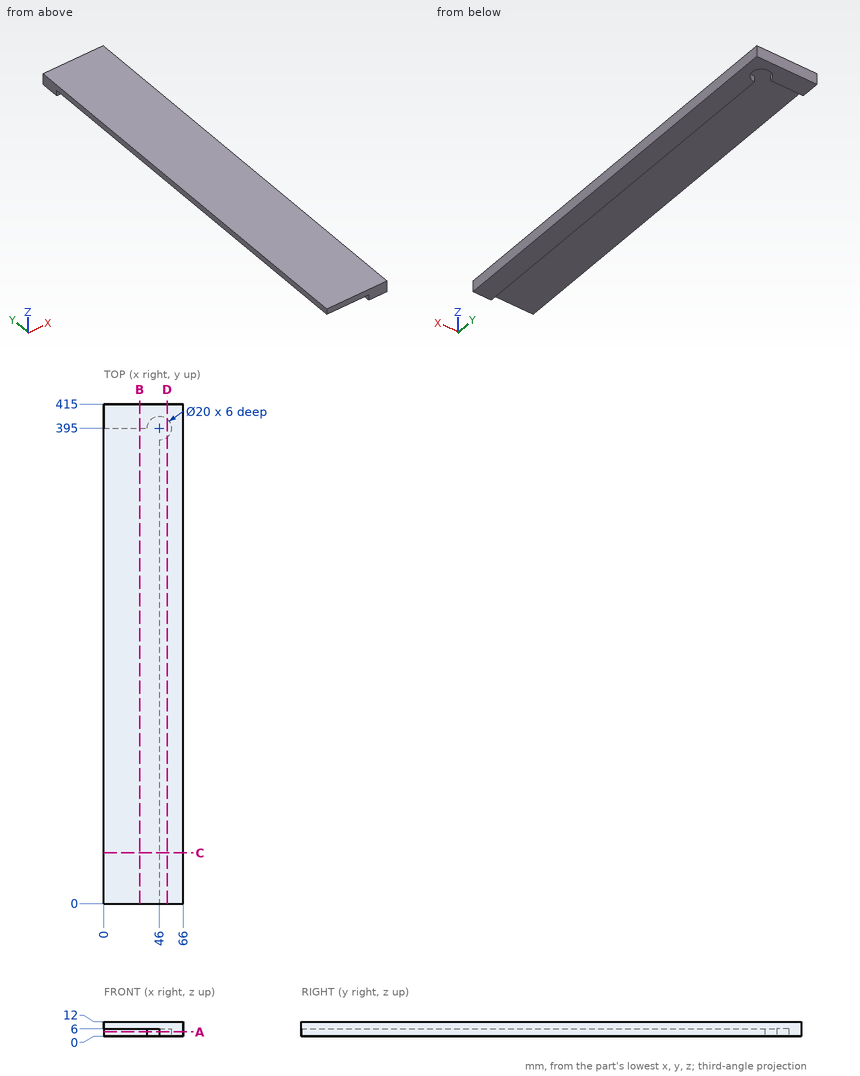
Answer from the drawing. Dimensions are ordinates in mm from the lowest x, y and z of the part. Coordinates: 2 decimals unless noted, no trailing zeros. Loops run counter-clockwise (first coordinate to the right, second up) from the corner with the lowest first, then second, coordinate; pieces in that order, holes last. Notation, with made-up numbers: (89.25, 19.5) -> (126.25, 19.5) arc R22 cw to (126.25, 33.5) -> close; hole circle Ø3 at (76.5, -3). An arc over 180 degrees is marked (long way). Answer as CSV lines item,"result".
Q1. The part is cut by section B-B on x = 29.5. Write down the section's boundary in (y, z), and give its area (3 significant figures).
Findings:
outline,"(0, 6) -> (395, 6) -> (395, 0) -> (415, 0) -> (415, 12) -> (0, 12) -> close"
area,"2,610 mm²"
Q2. Find the intervals of material crossed by probe 1 along X at (y, z) = (171, 3.75); probe 2 along Z at (x, y) = (45, 150); probe 3 along Y at (x, z) = (14.5, 1), in increasing order.
Findings:
probe 1,"x = 46 to 66"
probe 2,"z = 6 to 12"
probe 3,"y = 395 to 415"
Q3. The part is cut by section D-D on x = 52.5. Write down the section's boundary in (y, z).
Findings:
outline,"(0, 0) -> (387.4, 0) -> (387.4, 6) -> (402.6, 6) -> (402.6, 0) -> (415, 0) -> (415, 12) -> (0, 12) -> close"
Q4. Each of these flat-tipped pins is pushed along its axis until it touches: pin 1 (5 mm diameter, centred on y = 221.5, z = 3, fed in from -X); pin 2 (2 mm diameter, centred on x = 15.5, y = 41.5, fed in from -Z); pin 3 (1.8 mm diameter, centred on x = 9, z = 2.5, fed in from -Y). Where does it stop, or does it pass through?
Findings:
pin 1,"stops at x = 46"
pin 2,"stops at z = 6"
pin 3,"stops at y = 395"
Q5. The part is cut by section A-A on z = 3.5. Write down the section's boundary in (x, y).
Findings:
outline,"(0, 395) -> (36, 395) arc R10 cw (long way) to (46, 385) -> (46, 0) -> (66, 0) -> (66, 415) -> (0, 415) -> close"
Q6. The part is cut by section C-C on y = 42. Write down the section's boundary in (x, z), and give its area (3 significant figures).
Findings:
outline,"(0, 6) -> (46, 6) -> (46, 0) -> (66, 0) -> (66, 12) -> (0, 12) -> close"
area,"516 mm²"
